from build123d import *

# Parameters (mm, degrees)
SKETCH001_R        = 2.05
POCKET_DEPTH       = 98.592026
POLARPATTERN_COUNT = 6
PAD_DEPTH          = 5


with BuildPart() as part:
    # Sketch → Revolution (revolve)
    with BuildSketch(Plane.XY):
        with BuildLine():
            Line((-2.5, 2.5), (-2.5, -2.5))
            Line((-2.5, -2.5), (-16.45, -2.5))
            Line((-16.45, -2.5), (-16.45, -1.5))
            ThreePointArc((-16.45, -1.5), (-14.95, 0), (-16.45, 1.5))
            Line((-16.45, 1.5), (-16.45, 2.5))
            Line((-16.45, 2.5), (-2.5, 2.5))
        make_face()
    revolve(axis=Axis((0, 0, 0), (0, 1, 0)))

    # Sketch001 → Pocket (cut, through all)
    with BuildSketch(Plane.XZ.offset(2.5)):
        with Locations((0, 10)):
            Circle(SKETCH001_R)
    pocket = extrude(amount=-POCKET_DEPTH, mode=Mode.SUBTRACT)

    # PolarPattern: Pocket ×6 about axis
    polarpattern_axis = Axis((0, -2.5, 0), (0, -1, 0))
    for i in range(1, POLARPATTERN_COUNT):
        add(pocket.rotate(polarpattern_axis, i * 360 / POLARPATTERN_COUNT), mode=Mode.SUBTRACT)

    # Sketch002 → Pad (new body)
    with BuildSketch(Plane.XZ.offset(2.5)):
        with BuildLine():
            Line((-2, 1.5), (2, 1.5))
            ThreePointArc((2, 1.5), (0, 2.5), (-2, 1.5))
        make_face()
        with BuildLine():
            Line((2, -1.5), (-2, -1.5))
            ThreePointArc((-2, -1.5), (0, -2.5), (2, -1.5))
        make_face()
    extrude(amount=-PAD_DEPTH)


solid = part.part
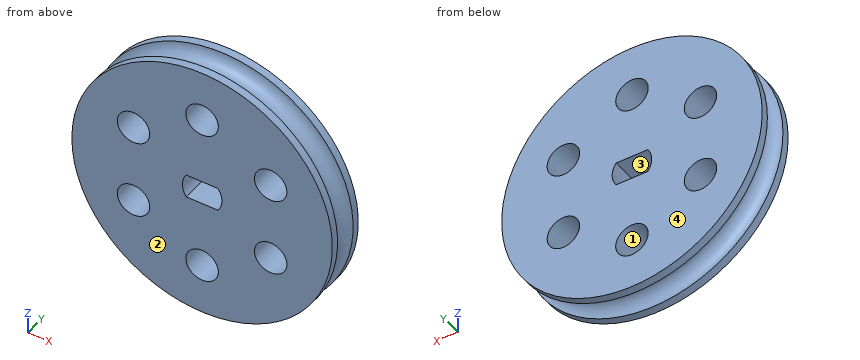
Here's how the part is built. I have some questions about the finished solid (model axes, mm). Face numbers are marked on the shaded views. A direction names the side the tool comes from. Round coordinates to 2 decimals unless told otherwise and drop trailing zeros. Order: outer loops, then holes, each group sorted by start corner. A loop starts at its lowest first (then second) coordinate and runs counter-clockwise, first axis right, second up. Notation, with made-up numbers: M 52,36 L 85,36 A8 cw 85,41 Z; hole C 1,44.25 d10. An arc over 180 degrees is marked long. One line per question, with ' | ' between items.
1) On a 3-axis mill with a long thin cutter (end or side, diameter ignored), from which of +Z, -Z, +X, -X, +Y, -Y can I reach the whole of each face in a straight line? I mean the marked faces 3 and 4. Say none if no direction works.
Checked values:
face 3: +Y, -Y | face 4: +Z, -Z, +X, -X, +Y
2) I need wall thicknesses on line 1 (Z direction, x = 0, y = -0.4); line 2 (Z direction, x = -7, y = -2.3); line 3 (Z direction, x = 0, y = -0.8). Which ranges of each line are inside material? Lowest first, please.
Checked values:
line 1: z = -15 to -12.05, -7.95 to -1.5, 1.5 to 7.95, 12.05 to 15 | line 2: z = -14.89 to -6.2, -3.8 to 3.8, 6.2 to 14.89 | line 3: z = -15.18 to -12.05, -7.95 to -1.5, 1.5 to 7.95, 12.05 to 15.18
3) We'd pull the mould along Z, two halves only. Please class the marked faces 1 and 2: released by +Z, released by -Z, zero draft, split by the parting line, or undercut.
Checked values:
face 1: undercut | face 2: zero draft
4) Imagine slicing it at A-A, the plane x = 0. Write out the boundary of the cut face in (y, z), plus the area to 3 significant figures.
Checked values:
outline: M -2.5,-16.45 L -1.5,-16.45 A1.5 cw 1.5,-16.45 L 2.5,-16.45 L 2.5,-12.05 L -2.5,-12.05 Z; M -2.5,-7.95 L 2.5,-7.95 L 2.5,-1.5 L -2.5,-1.5 Z; M -2.5,1.5 L 2.5,1.5 L 2.5,7.95 L -2.5,7.95 Z; M -2.5,12.05 L 2.5,12.05 L 2.5,16.45 L 1.5,16.45 A1.5 cw -1.5,16.45 L -2.5,16.45 Z | area: 101 mm²
5) Imagine slicing it at B-B, the plane y = -0.5. Write out the boundary of the cut face in (x, z), plus the area to 3 significant figures.
Checked values:
outline: C 0,0 d30.07; hole C -8.66,-5 d4.1; hole C -8.66,5 d4.1; hole C 0,-10 d4.1; hole C 0,10 d4.1; hole M -2,-1.5 L 2,-1.5 A2.5 ccw 2,1.5 L -2,1.5 A2.5 ccw Z; hole C 8.66,-5 d4.1; hole C 8.66,5 d4.1 | area: 617 mm²
6) I'm going to push flat-ended pins straight in: pin 1 Ø1.2 at (x, y) = (1, 0.5) entering from -Z; pin 2 Ø2 at (y, z) = (-1, -9) entering from +X. Where does each tip first touch, or does it pass through?
Checked values:
pin 1: stops at z = -15.4 | pin 2: stops at x = 14.3
7) Imagine slicing it at C-C, the plane x = 7. Count the separate pieces of the cut face and the enclosed holes in it, plus the area to 3 significant figures.
Checked values:
separate pieces: 3 | enclosed holes: 0 | area: 117 mm²
